Answer from the drawing. Dimensions are ordinates in mm from the lowest x, y and z of the part. A direction names the side the tool comes from. Coordinates: 2 decimals unless noted, no trailing zeros. Write each loop counter-clockwise with the first axis right and the second up, starting at its lowest first coordinate (ties: lowest second). Pieces come first, ordered by that corner, then holes. Notation, with made-up numbers: (39.25, 7.25) - (61.25, 7.25) arc R14 ccw to (61.25, 33.25) - close; hole circle Ø11 at (20, -0.75). An arc over 180 degrees is marked (long way). Use one line per item in the form item = value. Start each with the question number.
Item 1: For the marked faces 1, 2 and 3, determine the directions among +Z, -Z, +X, -X, +Y, -Y from which every point of the face is accessible in a straight line to the end or side of a thin tool.
Item 2: A cutting plane is placed at B-B (x = 20). Write down the section's boundary in (y, z).
Item 3: Determine the mould class of the marked faces 4, 5 and 6 for opening direction X: released by +X, released by -X, zero draft, split by the parting line, or undercut.
Item 4: A cutting plane is placed at D-D (x = 38.5). Write down the section's boundary in (y, z).
Item 5: A cutting plane is placed at A-A (y = 9). Write down the section's boundary in (x, z).
Item 6: Given pin 1 (1 mm diameter, centred on x = 30.5, z = 3, fed in from -Y); pin 2 (0.9 mm diameter, centred on x = 27.5, z = 1.5, fed in from -Y); pin 3 (2.5 mm diameter, centred on y = 2, z = 2, fed in from +X), each flat-ended and moving along its own axis, determine where each tip first touches the part or whether it passes through.
Item 7: Consider probe 1 along X at (y, z) = (31.5, 1.6); probe 2 along X at (y, z) = (13.5, 1.85); probe 3 along Y at (x, z) = (32, 4.4). Determine where each line is inside the solid, lowest interval first.
Item 8: A cutting plane is placed at C-C (z = 1.55). Write down the section's boundary in (x, y).
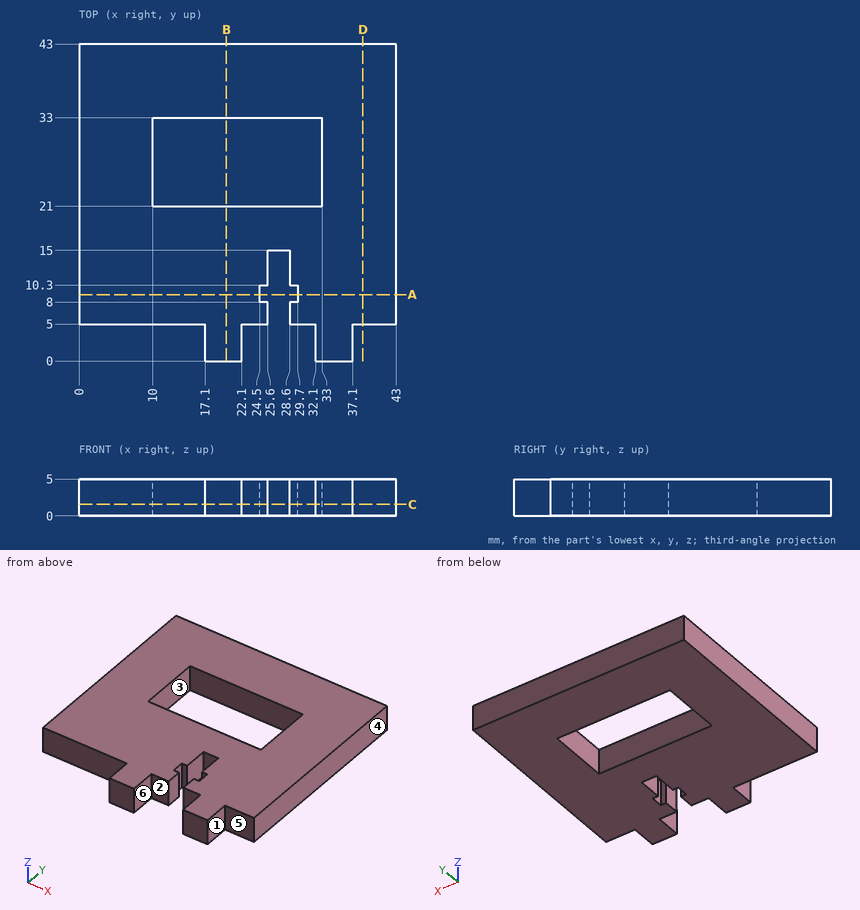
Answer:
q1.face_1 = +Z, -Z, +X, -Y
q1.face_2 = +Z, -Z, -Y
q1.face_3 = +Z, -Z
q2.outline = (0, 0) - (21, 0) - (21, 5) - (0, 5) - close; (33, 0) - (43, 0) - (43, 5) - (33, 5) - close
q3.face_4 = released by +X
q3.face_5 = zero draft
q3.face_6 = undercut
q4.outline = (5, 0) - (43, 0) - (43, 5) - (5, 5) - close
q5.outline = (0, 0) - (24.5, 0) - (24.5, 5) - (0, 5) - close; (29.7, 0) - (43, 0) - (43, 5) - (29.7, 5) - close
q6.pin_1 = 5
q6.pin_2 = 15
q6.pin_3 = 37.1
q7.probe_1 = 0 to 10, 33 to 43
q7.probe_2 = 0 to 25.6, 28.6 to 43
q7.probe_3 = 5 to 21, 33 to 43
q8.outline = (0, 5) - (17.1, 5) - (17.1, 0) - (22.1, 0) - (22.1, 5) - (25.6, 5) - (25.6, 8) - (24.5, 8) - (24.5, 10.3) - (25.6, 10.3) - (25.6, 15) - (28.6, 15) - (28.6, 10.3) - (29.7, 10.3) - (29.7, 8) - (28.6, 8) - (28.6, 5) - (32.1, 5) - (32.1, 0) - (37.1, 0) - (37.1, 5) - (43, 5) - (43, 43) - (0, 43) - close; hole (10, 21) - (33, 21) - (33, 33) - (10, 33) - close
